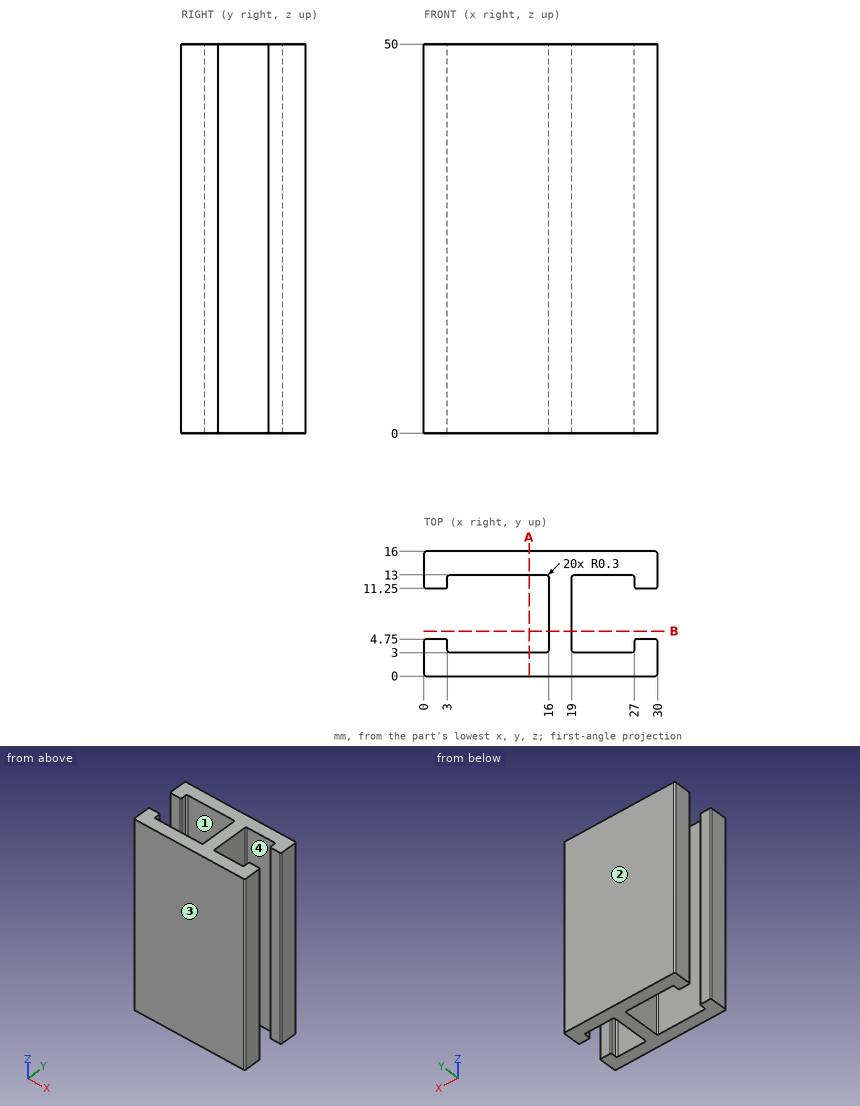
Here's the drawing with two shaded views (mm, measured from the low corner). I have some questions. A direction names the side the tool comes from. Coordinates: 2 decimals unless noted, no trailing zeros. Loops run counter-clockwise (first coordinate to the right, second up) from the corner with the lowest first, then second, coordinate; pieces in that order, holes last.
Item 1: Which directions (+Z, -Z, +X, -X, +Y, -Y) give clear straight access to the entire face, cutting with the end or side of a thin tool? Please do the marked faces 3 and 4.
Answers below:
face 3: +Z, -Z, +X, -X, -Y
face 4: +Z, -Z
Item 2: I'm going to push flat-ended pins straight in: pin 1 (1.5 mm diameter, centred on x = 5, z = 37, fed in from -Y); pin 2 (4.5 mm diameter, centred on y = 8, z = 36.5, fed in from -X). Where does each tip first touch, or does it pass through?
Answers below:
pin 1: stops at y = 0
pin 2: stops at x = 16
Item 3: Suppose I cut it at B-B (y = 5.75). Please give me the cut outline in (x, z).
Answers below:
outline: (16, 0) - (19, 0) - (19, 50) - (16, 50) - close
Item 4: Suppose I cut it at A-A (x = 13.5). Please give me the cut outline in (y, z), then the cut area to 3 significant figures.
Answers below:
outline: (0, 0) - (3, 0) - (3, 50) - (0, 50) - close; (13, 0) - (16, 0) - (16, 50) - (13, 50) - close
area: 300 mm2
Item 5: If we mould it in two halves opening along X, with no side actions, what happens to the marked faces 1 and 2? For each: released by +X, released by -X, zero draft, split by the parting line, or undercut.
Answers below:
face 1: undercut
face 2: zero draft
Item 6: Please list where these lines run through material, in increasing order: L1, parallel to X at y = 12.25, z = 11; L2, parallel to Y at x = 12.5, z = 6.5; L3, parallel to Y at x = 28.5, z = 16.5.
Answers below:
L1: x = 0 to 3, 16 to 19, 27 to 30
L2: y = 0 to 3, 13 to 16
L3: y = 0 to 4.75, 11.25 to 16
